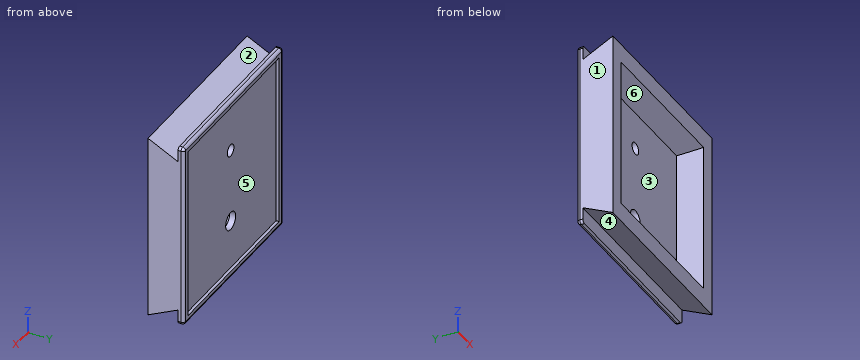
```python
from build123d import *

# Parameters (mm, degrees)
SKETCH1_W           = 60
SKETCH1_H           = 62.5
BOSS_EXTRUDE1_DEPTH = 10
CUT_EXTRUDE1_DEPTH  = 69.385396833
CUT_EXTRUDE2_DEPTH  = 69.385396833
SKETCH4_W           = 60
SKETCH4_H           = 62.5
BOSS_EXTRUDE2_DEPTH = 2
FILLET1_R           = 1
FILLET2_R           = 1
SKETCH5_W           = 55
SKETCH5_H           = 58
CUT_EXTRUDE3_DEPTH  = 1
SKETCH6_W           = 50
SKETCH6_H           = 50
CUT_EXTRUDE4_DEPTH  = 9
SKETCH7_R           = 3
CUT_EXTRUDE5_DEPTH  = 9
SKETCH8_R           = 2
CUT_EXTRUDE6_DEPTH  = 10


with BuildPart() as part:
    # Sketch1 → Boss-Extrude1 (new body)
    with BuildSketch(Plane(origin=(0, 0, 0), x_dir=(1, 0, 0), z_dir=(0, 1, 0))):
        Rectangle(SKETCH1_W, SKETCH1_H)
    extrude(amount=BOSS_EXTRUDE1_DEPTH)

    # Sketch2 → Cut-Extrude1 (cut, through all)
    with BuildSketch(Plane(origin=(30, 0, 0), x_dir=(0, 0, -1), z_dir=(1, 0, 0))):
        Polygon((31.25, 0), (26.25, 10), (31.25, 10), align=None)
    extrude(amount=-CUT_EXTRUDE1_DEPTH, mode=Mode.SUBTRACT)

    # Sketch3 → Cut-Extrude2 (cut, through all)
    with BuildSketch(Plane(origin=(30, 0, 0), x_dir=(0, 0, -1), z_dir=(1, 0, 0))):
        Polygon((-31.25, 0), (-26.25, 10), (-31.25, 10), align=None)
    extrude(amount=-CUT_EXTRUDE2_DEPTH, mode=Mode.SUBTRACT)

    # Sketch4 → Boss-Extrude2 (add)
    with BuildSketch(Plane(origin=(0, 10, 0), x_dir=(1, 0, 0), z_dir=(0, 1, 0))):
        Rectangle(SKETCH4_W, SKETCH4_H)
    extrude(amount=BOSS_EXTRUDE2_DEPTH)

    # Fillet1
    fillet1_edges = [part.edges().sort_by_distance(p)[0] for p in [
        (-30, 11, 31.25),
        (30, 11, 31.25),
        (30, 11, -31.25),
        (-30, 11, -31.25),
    ]]
    fillet(fillet1_edges, radius=FILLET1_R)

    # Fillet2
    fillet2_edges = [part.edges().sort_by_distance(p)[0] for p in [
        (0, 12, -31.25),
        (30, 12, 0),
        (0, 12, 31.25),
        (-30, 12, 0),
        (29.707106781, 12, 30.957106781),
        (-29.707106781, 12, 30.957106781),
        (-29.707106781, 12, -30.957106781),
        (29.707106781, 12, -30.957106781),
    ]]
    fillet(fillet2_edges, radius=FILLET2_R)

    # Sketch5 → Cut-Extrude3 (cut)
    with BuildSketch(Plane(origin=(0, 12, 0), x_dir=(1, 0, 0), z_dir=(0, 1, 0))):
        Rectangle(SKETCH5_W, SKETCH5_H)
    extrude(amount=-CUT_EXTRUDE3_DEPTH, mode=Mode.SUBTRACT)

    # Sketch6 → Cut-Extrude4 (cut)
    with BuildSketch(Plane.XZ):
        Rectangle(SKETCH6_W, SKETCH6_H)
    extrude(amount=-CUT_EXTRUDE4_DEPTH, mode=Mode.SUBTRACT)

    # Sketch7 → Cut-Extrude5 (cut)
    with BuildSketch(Plane.XZ.offset(-9)):
        with Locations(Location((0, -12.5, 0), (0, 0, 270))):
            Circle(SKETCH7_R)
    extrude(amount=-CUT_EXTRUDE5_DEPTH, mode=Mode.SUBTRACT)

    # Sketch8 → Cut-Extrude6 (cut)
    with BuildSketch(Plane(origin=(0, 11, 0), x_dir=(1, 0, 0), z_dir=(0, 1, 0))):
        with Locations(Location((0, -12.5, 0), (0, 0, 270))):
            Circle(SKETCH8_R)
    extrude(amount=-CUT_EXTRUDE6_DEPTH, mode=Mode.SUBTRACT)


solid = part.part
```
Geometry: final body of the model. Coordinates: model frame, mm. Face numbers are marked on the shaded views. A direction names the side the tool comes from. Round coordinates to 2 decimals unless told otherwise and drop trailing zeros. Order: outer loops, then holes, each group sorted by start corner. A loop starts at its lowest first (then second) coordinate and runs counter-clockwise, first axis right, second up. Notation, with made-up numbers: (55.5, 59) -> (102.5, 59) arc R20 cw to (102.5, 65) -> close; hole circle Ø2 at (7, 68). An arc over 180 degrees is marked (long way). Use one line per item in the form item = value. Start each with the question number.
1. Cut plane C-C (x = 0). Return the cut outline in (y, z).
2. Cut plane B-B (y = 7). Return the cut outline in (x, z).
3. Pin query (flat end, axial travel): pin 1 Ø1.1 at (x, y) = (-13, 11.5) entering from +Z; pin 2 Ø0.8 at (y, z) = (11.5, -10) entering from -X (3 decimals); pin 3 Ø7 at (x, z) = (0, -12.5) entering from -Y; pin 4 Ø2 at (x, y) = (22, 6) entering from -Z. Return the tip coordinate at first contact, or that it passes through.
4. Draft query along Y for the marked faces 4, 5 and 6. Return one class per face: pulls with the +Y half, pulls with the -Y half, needs draft (parallel to the pull), parting line crosses it, or undercut.
5. Reachability of the marked faces 1, 2 and 3 from +Z, -Z, +X, -X, +Y, -Y: full face, straight path, thin tool, end or side. Return the list, or none.
6. Line query: probe 1 along X at (y, z) = (9.55, -12.5); probe 2 along X at (y, z) = (5, 10.5); probe 3 along Y at (x, z) = (-15, -14). Output: solid intervals per line, ascending.
7. Cut plane D-D (z = 0). Return the cut outline in (x, y), then the cut area to 3 significant figures.
8. Cut plane A-A (z = -12.5). Return the cut outline in (x, y).
Solution:
q1.outline = (0, -31.25) -> (10, -26.25) -> (10, -31.25) -> (11, -31.25) arc R1 ccw to (12, -30.25) -> (12, -29) -> (11, -29) -> (11, -15.5) -> (9, -15.5) -> (9, -25) -> (0, -25) -> close; (0, 25) -> (9, 25) -> (9, 14.5) -> (11, 14.5) -> (11, 29) -> (12, 29) -> (12, 30.25) arc R1 ccw to (11, 31.25) -> (10, 31.25) -> (10, 26.25) -> (0, 31.25) -> close; (9, -9.5) -> (11, -9.5) -> (11, 10.5) -> (9, 10.5) -> close
q2.outline = (-30, -27.75) -> (30, -27.75) -> (30, 27.75) -> (-30, 27.75) -> close; hole (-25, -25) -> (25, -25) -> (25, 25) -> (-25, 25) -> close
q3.pin_1 = 31.25
q3.pin_2 = -29.995
q3.pin_3 = 9
q3.pin_4 = -28.75
q4.face_4 = undercut
q4.face_5 = pulls with the +Y half
q4.face_6 = needs draft
q5.face_1 = +Z, -Z, -X, +Y, -Y
q5.face_2 = +Z, +X, -X
q5.face_3 = -Y
q6.probe_1 = -30 to -3, 3 to 30
q6.probe_2 = -30 to -25, 25 to 30
q6.probe_3 = 9 to 11
q7.outline = (-30, 0) -> (-25, 0) -> (-25, 9) -> (25, 9) -> (25, 0) -> (30, 0) -> (30, 11) arc R1 ccw to (29, 12) -> (27.5, 12) -> (27.5, 11) -> (-27.5, 11) -> (-27.5, 12) -> (-29, 12) arc R1 ccw to (-30, 11) -> close
q7.area = 215 mm^2
q8.outline = (-30, 0) -> (-25, 0) -> (-25, 9) -> (-3, 9) -> (-3, 11) -> (-27.5, 11) -> (-27.5, 12) -> (-29, 12) arc R1 ccw to (-30, 11) -> close; (3, 9) -> (25, 9) -> (25, 0) -> (30, 0) -> (30, 11) arc R1 ccw to (29, 12) -> (27.5, 12) -> (27.5, 11) -> (3, 11) -> close
